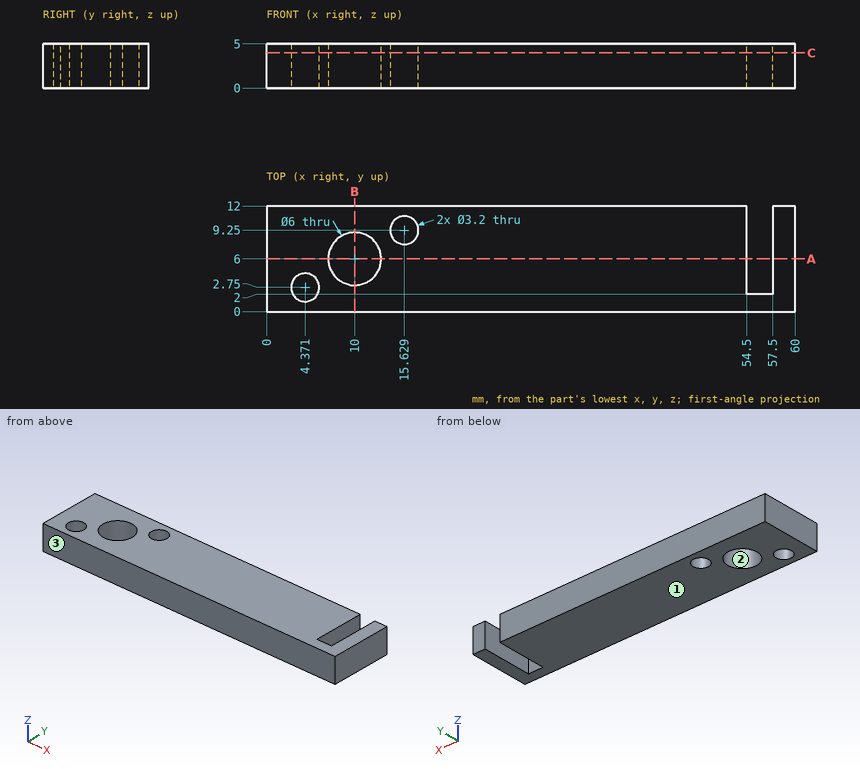
The drawing under review shows one solid part. Ordinate dimensions are in mm from its lowest x, y, z. Round coordinates to 2 decimals unless told otherwise and drop trailing zeros. Order: outer loops, then holes, each group sorted by start corner. A loop starts at its lowest first (then second) coordinate and runs counter-clockwise, first axis right, second up. Notation, with made-up numbers: M 0.5,69 L 24.5,69 A14 ccw 24.5,91 Z; hole C -21,72.25 d11. An arc over 180 degrees is marked long. Answer as CSV lines item,"result". Start each with the question number.
1) Add section B-B (x = 10). Give the boundary of the cut face in (y, z).
2) For pin 1 Ø1.5 at (x, z) = (56, 2.5) entering from +Y; pin 2 Ø3.5 at (x, y) = (10, 6) entering from -Z, all flat-tipped, find the tip position at first contact; note any pin that passes through.
3) The part is to be moulded in two halves that separate along Y. For the marked faces 1, 2 and 3, say which applies: +Y half, -Y half, draft (parallel to the pull), parting line (faces both ways), or undercut.
4) Add section A-A (y = 6). Give the boundary of the cut face in (x, z).
5) Add section C-C (z = 4). Give the boundary of the cut face in (x, y), then the cut area to 3 significant figures.
6) Wall thickness on line 1 along X through (y, z) = (4.75, 1.15); line 2 along X through (y, z) = (7.5, 0.7); line 3 along X through (y, z) = (11, 3.45): over which ranges is each line inside the solid? List them lowest first. Write a range as [from, to].
Resolved:
1,outline,"M 0,0 L 3,0 L 3,5 L 0,5 Z; M 9,0 L 12,0 L 12,5 L 9,5 Z"
2,pin 1,"y = 2"
2,pin 2,"through"
3,face 1,"draft"
3,face 2,"undercut"
3,face 3,"-Y half"
4,outline,"M 0,0 L 7,0 L 7,5 L 0,5 Z; M 13,0 L 54.5,0 L 54.5,5 L 13,5 Z; M 57.5,0 L 60,0 L 60,5 L 57.5,5 Z"
5,outline,"M 0,0 L 60,0 L 60,12 L 57.5,12 L 57.5,2 L 54.5,2 L 54.5,12 L 0,12 Z; hole C 4.37,2.75 d3.2; hole C 10,6 d6; hole C 15.63,9.25 d3.2"
5,area,"646 mm^2"
6,line 1,"[0, 7.27], [12.73, 54.5], [57.5, 60]"
6,line 2,"[0, 7.4], [12.6, 54.5], [57.5, 60]"
6,line 3,"[0, 54.5], [57.5, 60]"
